Could you check a few things on this model? Use its own coordinates, in mm. Face numbers are marked on the shaded views. A direction names the side the tool comes from. Round coordinates to 2 decimals unless told otherwise and drop trailing zeros. Order: outer loops, then holes, each group sorted by start corner. A loop starts at its lowest first (then second) coordinate and runs counter-clockwise, first axis right, second up. Notation, with made-up numbers: (25, -1.5) -> (64, -1.5) arc R26 cw to (64, 35.5) -> close; hole circle Ø3 at (26.25, 75.5). An arc over 180 degrees is marked (long way). Put each result on its own line as item: value. Start each with the question number.
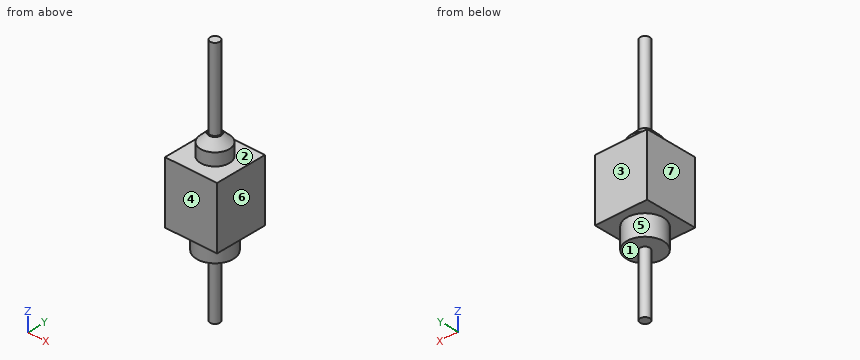
from build123d import *

# Parameters (mm, degrees)
SKETCH1_W           = 2.54
SKETCH1_H           = 2.54
BOSS_EXTRUDE1_DEPTH = 3
SKETCH2_R           = 0.23
BOSS_EXTRUDE2_DEPTH = 4
SKETCH3_R           = 0.89
BOSS_EXTRUDE3_DEPTH = 1
SKETCH4_R           = 0.23
BOSS_EXTRUDE4_DEPTH = 4.96
SKETCH5_R           = 0.7
BOSS_EXTRUDE5_DEPTH = 1
CHAMFER1_SIZE       = 0.4


with BuildPart() as part:
    # Sketch1 → Boss-Extrude1 (new body)
    with BuildSketch(Plane.XY):
        Rectangle(SKETCH1_W, SKETCH1_H)
    extrude(amount=BOSS_EXTRUDE1_DEPTH)

    # Sketch2 → Boss-Extrude2 (add)
    with BuildSketch(Plane(origin=(0, 0, 0), x_dir=(-1, 0, 0), z_dir=(0, 0, -1))):
        Circle(SKETCH2_R)
    extrude(amount=BOSS_EXTRUDE2_DEPTH)

    # Sketch3 → Boss-Extrude3 (add)
    with BuildSketch(Plane(origin=(0, 0, 0), x_dir=(-1, 0, 0), z_dir=(0, 0, -1))):
        Circle(SKETCH3_R)
    extrude(amount=BOSS_EXTRUDE3_DEPTH)

    # Sketch4 → Boss-Extrude4 (add)
    with BuildSketch(Plane.XY.offset(3)):
        Circle(SKETCH4_R)
    extrude(amount=BOSS_EXTRUDE4_DEPTH)

    # Sketch5 → Boss-Extrude5 (add)
    with BuildSketch(Plane.XY.offset(3)):
        Circle(SKETCH5_R)
    extrude(amount=BOSS_EXTRUDE5_DEPTH)

    # Chamfer1
    chamfer1_edges = [part.edges().sort_by_distance(p)[0] for p in [
        (-0.7, 0, 4),
    ]]
    chamfer(chamfer1_edges, length=CHAMFER1_SIZE)


solid = part.part
1. Which directions (+Z, -Z, +X, -X, +Y, -Y) give clear straight access to the entire face, cutting with the end or side of a thin tool? Please do the marked faces 1, 2 and 3.
2. If we section it at A-A, the plane y = 0: Please give me the cut outline in (x, z).
3. If we section it at C-C, the plane z = 5.75: Please give me the cut outline in (x, y), then the cut area to 3 significant figures.
4. If we section it at D-D, the plane y = -1: Please give me the cut outline in (x, z), then the cut area to 3 significant figures.
5. Thinking about a two-plate mould opening in X: for the marked faces 4, 5, 6 and 7, which applies, +X half, -X half, draft (parallel to the pull), parting line (faces both ways), or undercut?
6. For pin 1 Ø0.8 at (x, y) = (0.5, 0) entering from +Z, with a flat end and sliding along its axis, tell me the tip position at first contact or that it passes through.
7. I need wall thicknesses on L1, parallel to Z at x = 0.55, y = 1.05; L2, parallel to Z at x = -0.6, y = 0.5; L3, parallel to Y at x = -0.1, z = 6. Which ranges of each line are inside material? Lowest first, please.
Results below:
1. face 1: -Z
1. face 2: +Z
1. face 3: +Z, -Z, +X, -X, +Y
2. outline: (-1.27, 0) -> (-0.89, 0) -> (-0.89, -1) -> (-0.23, -1) -> (-0.23, -4) -> (0.23, -4) -> (0.23, -1) -> (0.89, -1) -> (0.89, 0) -> (1.27, 0) -> (1.27, 3) -> (0.7, 3) -> (0.7, 3.6) -> (0.3, 4) -> (0.23, 4) -> (0.23, 7.96) -> (-0.23, 7.96) -> (-0.23, 4) -> (-0.3, 4) -> (-0.7, 3.6) -> (-0.7, 3) -> (-1.27, 3) -> close
3. outline: circle Ø0.46 at (0, 0)
3. area: 0.166 mm2
4. outline: (-1.27, 0) -> (1.27, 0) -> (1.27, 3) -> (-1.27, 3) -> close
4. area: 7.62 mm2
5. face 4: draft
5. face 5: parting line
5. face 6: +X half
5. face 7: -X half
6. pin 1: z = 7.96
7. L1: 0 to 3
7. L2: -1 to 3
7. L3: -0.21 to 0.21
